```python
from build123d import *

# Parameters (mm, degrees)
F0_R     = 86
F0_R_2   = 81
F1_DEPTH = 3
F2_DEPTH = 50
F3_T     = -2
F4_R     = 1.6
F4_W     = 38
F4_H     = 14
F5_DEPTH = 2


with BuildPart() as f1:
    # F0 (on Top) → F1 (new body)
    with BuildSketch(Plane.XY):
        Circle(F0_R)
        Circle(F0_R_2, mode=Mode.SUBTRACT)
        Circle(F0_R_2)
    extrude(amount=F1_DEPTH)

    # F0 (on Top) → F2 (join)
    with BuildSketch(Plane.XY):
        Circle(F0_R_2)
    extrude(amount=F2_DEPTH)

    # F3
    f3_openings = [f1.faces().sort_by_distance(p)[0] for p in [
        (0, 0, 50),
    ]]
    offset(amount=F3_T, openings=f3_openings, kind=Kind.INTERSECTION)

    # F4 (on face) → F5 (cut)
    with BuildSketch(Plane(origin=(0, 0, 0), x_dir=(1, 0, 0), z_dir=(0, 0, -1))):
        with Locations((0, 19.0525588833)):
            Circle(F4_R)
        with Locations((0, 0.9737205584)):
            Rectangle(F4_W, F4_H)
        with Locations((16.5, -9.5262794416)):
            Circle(F4_R)
        with Locations((-16.5, -9.5262794416)):
            Circle(F4_R)
    extrude(amount=-F5_DEPTH, mode=Mode.SUBTRACT)


solid = f1.part
```
Verification items for the finished model (mm, model axes). A direction names the side the tool comes from. Give positions to 0.01 mm unless a question says otherwise; leave off trailing zeros. Loops run counter-clockwise (first coordinate to the right, second up) from the corner with the lowest first, then second, coordinate; pieces in that order, holes last.
1. Section check D-D, the plane y = 72. Enter the section's corners in (x, z).
2. Set-up check for faces 4 (the cylindrical face through (43.545, 68.3, 26.171)), 5 (the flat face through (-20, 1, 0)): record each of +Z, -Z, +X, -X, +Y, -Y from which the full face is reachable in a straight line by a thin tool's end or side.
3. Thickness scan on line 1 (Y direction, x = 0, z = 1.6); line 2 (X direction, y = 1.5, z = 5.5); line 3 (Y direction, x = 0, z = 12). Record the ranges inside material, lowest first.
4. Section check B-B, the plane x = 28.5. Enter the section's corners in (y, z).
5. Section check A-A, the plane y = 0. Enter the section's corners in (x, z), then the cut area to 3 significant figures.
6. Section check C-C, the plane z = 24. Enter the section's corners in (x, y), then the cut area to 3 significant figures.
7. Go/stop test with flat-tipped pins: pin 1 Ø8 at (y, z) = (49.5, 27.5) entering from -X; pin 2 Ø4 at (x, z) = (9, 43) entering from -Y; pin 3 Ø1 at (x, z) = (4.5, 1) entering from -Y; pin 4 Ø3 at (x, y) = (-16.5, 9.53) entering from -Z. Record where each tip stops, or that it passes through.
8. Mould release check, pull along X, two halves, no side actions. Record for faces 1 (the cylindrical face through (-58.23, 53.39, 25.66)), 2 (the cylindrical face through (-11.195, 85.268, 1.479)), 3 (the flat face through (-58, -57, 3)): released by +X, released by -X, zero draft, split by the parting line, or undercut.
Geometry says:
1. outline: (-47.03, 0) - (47.03, 0) - (47.03, 3) - (37.11, 3) - (37.11, 50) - (32.51, 50) - (32.51, 2) - (-32.51, 2) - (-32.51, 50) - (-37.11, 50) - (-37.11, 3) - (-47.03, 3) - close
2. face 4: +Z
2. face 5: -Z, +X, -X, +Y, -Y
3. line 1: y = -86 to -20.65, -17.45 to -7.97, 6.03 to 86
3. line 2: x = -80.99 to -78.99, 78.99 to 80.99
3. line 3: y = -81 to -79, 79 to 81
4. outline: (-81.14, 0) - (81.14, 0) - (81.14, 3) - (75.82, 3) - (75.82, 50) - (73.68, 50) - (73.68, 2) - (-73.68, 2) - (-73.68, 50) - (-75.82, 50) - (-75.82, 3) - (-81.14, 3) - close
5. outline: (-86, 0) - (-19, 0) - (-19, 2) - (-79, 2) - (-79, 50) - (-81, 50) - (-81, 3) - (-86, 3) - close; (19, 0) - (86, 0) - (86, 3) - (81, 3) - (81, 50) - (79, 50) - (79, 2) - (19, 2) - close
5. area: 470 mm2
6. outline: circle Ø162 at (0, 0); hole circle Ø158 at (0, 0)
6. area: 1,010 mm2
7. pin 1: stops at x = -67.01
7. pin 2: stops at y = -80.7
7. pin 3: stops at y = -85.91
7. pin 4: passes through
8. face 1: undercut
8. face 2: split by the parting line
8. face 3: zero draft
